Build history of the part. All positions in model axes, mm. Face numbers are marked on the shaded views. A direction names the side the tool comes from. Round coordinates to 2 decimals unless told otherwise and drop trailing zeros. Write each loop counter-clockwise with the first axis right and the second up, starting at its lowest first coordinate (ties: lowest second). Pieces come first, ordered by that corner, then holes. Notation, with made-up numbers: (-9, 12.5) -> (50, 12.5) arc R15 ccw to (50, 27.5) -> close; hole circle Ø9 at (57.25, 33.5). An arc over 180 degrees is marked (long way). Return JSON: item names as keys, results as strings.
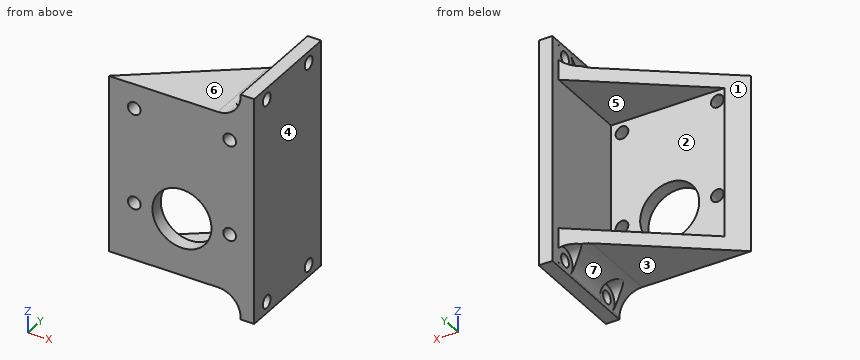
from build123d import *

# Parameters (mm, degrees)
EXTRUDE_1_DEPTH           = 39
SHELL_1_T                 = -3
SKETCH_2_R                = 1.4
CUT_EXTRUDE_1_DEPTH       = 30
SKETCH_3_R                = 6.5
CUT_EXTRUDE_2_DEPTH       = 5
SKETCH_5_W                = 50
SKETCH_5_H                = 24
EXTRUDE_2_DEPTH           = 3
SKETCH_4_R                = 1.4
CUT_EXTRUDE_3_DEPTH       = 5
FILLET_1_R                = 5
CUT_EXTRUDE_4_OUTLINE_R   = 1.4
CUT_EXTRUDE_4_OUTLINE_R_2 = 2.75
CUT_EXTRUDE_4_DEPTH       = 3.43874985


with BuildPart() as part:
    # ｽｹｯﾁ1 → ﾎﾞｽ - 押し出し1 (new body)
    with BuildSketch(Plane.XY):
        Polygon((0, 0), (32, 0), (32, 24), align=None)
    extrude(amount=EXTRUDE_1_DEPTH)

    # ｼｪﾙ1
    shell_1_openings = [part.faces().sort_by_distance(p)[0] for p in [
        (16, 12, 19.5),
    ]]
    offset(amount=SHELL_1_T, openings=shell_1_openings, kind=Kind.INTERSECTION)

    # ｽｹｯﾁ2 → ｶｯﾄ - 押し出し1 (cut)
    with BuildSketch(Plane.XZ):
        with Locations(Location((26.6, 12.609, 0), (0, 0, 270))):
            Circle(SKETCH_2_R)
        with Locations(Location((5.6, 12.609, 0), (0, 0, 270))):
            Circle(SKETCH_2_R)
        with Locations(Location((5.6, 33.609, 0), (0, 0, 270))):
            Circle(SKETCH_2_R)
        with Locations(Location((26.6, 33.609, 0), (0, 0, 270))):
            Circle(SKETCH_2_R)
    extrude(amount=-CUT_EXTRUDE_1_DEPTH, mode=Mode.SUBTRACT)

    # ｽｹｯﾁ3 → ｶｯﾄ - 押し出し2 (cut)
    with BuildSketch(Plane.XZ):
        with Locations(Location((16.1, 12.609, 0), (0, 0, 270))):
            Circle(SKETCH_3_R)
    extrude(amount=-CUT_EXTRUDE_2_DEPTH, mode=Mode.SUBTRACT)

    # ｽｹｯﾁ5 → ﾎﾞｽ - 押し出し2 (add)
    with BuildSketch(Plane(origin=(32, 0, 0), x_dir=(0, 0, -1), z_dir=(1, 0, 0))):
        with Locations((-19.5, 12)):
            Rectangle(SKETCH_5_W, SKETCH_5_H)
    extrude(amount=-EXTRUDE_2_DEPTH)

    # ｽｹｯﾁ4 → ｶｯﾄ - 押し出し3 (cut)
    with BuildSketch(Plane(origin=(32, 0, 0), x_dir=(0, 0, -1), z_dir=(1, 0, 0))):
        with Locations((3, 19.5)):
            Circle(SKETCH_4_R)
        with Locations((-42, 19.5)):
            Circle(SKETCH_4_R)
        with Locations((-42, 4.5)):
            Circle(SKETCH_4_R)
        with Locations((3, 4.5)):
            Circle(SKETCH_4_R)
    extrude(amount=-CUT_EXTRUDE_3_DEPTH, mode=Mode.SUBTRACT)

    # ﾌｨﾚｯﾄ1
    # the kernel refuses this fillet: 5 mm, written as the material it adds along each edge
    with BuildSketch(Plane(origin=(29, 34.25, 39), x_dir=(-1, 0, 0), z_dir=(0, -1, 0))) as fillet_1_piece_1_section:
        with BuildLine():
            CenterArc((FILLET_1_R, -FILLET_1_R), FILLET_1_R, 90, 90)
            Line((0, -FILLET_1_R), (0, 0))
            Line((0, 0), (FILLET_1_R, 0))
        make_face()
    fillet_1_piece_1 = extrude(amount=34.25, mode=Mode.PRIVATE)
    fillet_1_piece_1 = split(fillet_1_piece_1, bisect_by=Plane(origin=(35, 26.25, 39), z_dir=(0.6, -0.8, 0)), keep=Keep.TOP, mode=Mode.PRIVATE)
    fillet_1_piece_1 = fillet_1_piece_1 - Plane(origin=(29, 4.5, 42), x_dir=(0, 0, -1), z_dir=(1, 0, 0)) * Cylinder(1.4, 89, mode=Mode.PRIVATE)
    fillet_1_piece_1 = fillet_1_piece_1 - Plane(origin=(29, 19.5, 42), x_dir=(0, 0, -1), z_dir=(1, 0, 0)) * Cylinder(1.4, 89, mode=Mode.PRIVATE)
    add(fillet_1_piece_1)
    with BuildSketch(Plane(origin=(29, 34.25, 0), x_dir=(-1, 0, 0), z_dir=(0, -1, 0))) as fillet_1_piece_2_section:
        with BuildLine():
            CenterArc((FILLET_1_R, FILLET_1_R), FILLET_1_R, 180, 90)
            Line((0, FILLET_1_R), (0, 0))
            Line((0, 0), (FILLET_1_R, 0))
        make_face()
    fillet_1_piece_2 = extrude(amount=34.25, mode=Mode.PRIVATE)
    fillet_1_piece_2 = split(fillet_1_piece_2, bisect_by=Plane(origin=(35, 26.25, 0), z_dir=(0.6, -0.8, 0)), keep=Keep.TOP, mode=Mode.PRIVATE)
    fillet_1_piece_2 = fillet_1_piece_2 - Plane(origin=(29, 4.5, -3), x_dir=(0, 0, -1), z_dir=(1, 0, 0)) * Cylinder(1.4, 89, mode=Mode.PRIVATE)
    fillet_1_piece_2 = fillet_1_piece_2 - Plane(origin=(29, 19.5, -3), x_dir=(0, 0, -1), z_dir=(1, 0, 0)) * Cylinder(1.4, 89, mode=Mode.PRIVATE)
    add(fillet_1_piece_2)

    # ｶｯﾄ - 押し出し4: read off the stored shape, not the designer's step
    # ｶｯﾄ - 押し出し4 outline → ｶｯﾄ - 押し出し4 (cut)
    # profile 1 of 4: a face of its own
    with BuildSketch(Plane.ZY.offset(-29)):
        with BuildLine():
            ThreePointArc((44, 17.612541391), (44.75, 19.5), (44, 21.387458609))
            ThreePointArc((44, 21.387458609), (43.799721616, 21.579303274), (43.58113883, 21.75))
            ThreePointArc((43.58113883, 21.75), (42, 22.25), (40.41886117, 21.75))
            ThreePointArc((40.41886117, 21.75), (39.920696726, 17.700278384), (44, 17.612541391))
        make_face()
        with Locations((42, 19.5)):
            Circle(CUT_EXTRUDE_4_OUTLINE_R, mode=Mode.SUBTRACT)
    # profile 2 of 4: a face of its own
    with BuildSketch(Plane.ZY.offset(-29)):
        with BuildLine():
            ThreePointArc((44, 2.612541391), (44.75, 4.5), (44, 6.387458609))
            ThreePointArc((44, 6.387458609), (39.25, 4.5), (44, 2.612541391))
        make_face()
        with Locations((42, 4.5)):
            Circle(CUT_EXTRUDE_4_OUTLINE_R, mode=Mode.SUBTRACT)
    # profile 3 of 4: a face of its own
    with BuildSketch(Plane.ZY.offset(-29)):
        with BuildLine():
            ThreePointArc((-5, 21.387458609), (-1.200278384, 17.420696726), (-4.58113883, 21.75))
            ThreePointArc((-4.58113883, 21.75), (-4.799721616, 21.579303274), (-5, 21.387458609))
        make_face()
        with Locations((-3, 19.5)):
            Circle(CUT_EXTRUDE_4_OUTLINE_R, mode=Mode.SUBTRACT)
    # profile 4 of 4: a face of its own
    with BuildSketch(Plane.ZY.offset(-29)):
        with Locations((-3, 4.5)):
            Circle(CUT_EXTRUDE_4_OUTLINE_R_2)
        with Locations((-3, 4.5)):
            Circle(CUT_EXTRUDE_4_OUTLINE_R, mode=Mode.SUBTRACT)
    extrude(amount=CUT_EXTRUDE_4_DEPTH, mode=Mode.SUBTRACT)


solid = part.part
Q1. Saw through at C-C on z = 4. List the corners of the cut face in (x, y), then the cut area to 3 significant figures.
Verdict:
{"outline": "(0, 0) -> (32, 0) -> (32, 24) -> (29, 24) -> (29, 3) -> (4, 3) -> close", "area": "153 mm²"}
Q2. Saw through at D-D on y = 15. List the corners of the cut face in (x, z).
Verdict:
{"outline": "(20, 0) -> (24, 0) arc R5 cw to (29, -5) -> (29, -5.5) -> (32, -5.5) -> (32, 44.5) -> (29, 44.5) -> (29, 44) arc R5 cw to (24, 39) -> (20, 39) -> (20, 36) -> (29, 36) -> (29, 3) -> (20, 3) -> close"}
Q3. Saw through at B-B on y = 4.5. List the corners of the cut face in (x, z).
Verdict:
{"outline": "(6, 0) -> (24, 0) arc R5 cw to (25.56, -0.25) -> (29, -0.25) -> (29, -1.6) -> (32, -1.6) -> (32, 40.6) -> (29, 40.6) -> (29, 39.25) -> (25.56, 39.25) arc R5 cw to (24, 39) -> (6, 39) -> (6, 36) -> (29, 36) -> (29, 3) -> (6, 3) -> close; (29, -5.5) -> (32, -5.5) -> (32, -4.4) -> (29, -4.4) -> close; (29, 43.4) -> (32, 43.4) -> (32, 44.5) -> (29, 44.5) -> close"}
Q4. 3-axis set-ups, long thin cutter, end or side, ignore diameter. For the marked faces 1, 2 and 3: which of +Z, -Z, +X, -X, +Y, -Y reach the whole face in a straight line?
Verdict:
{"face 1": "+Z, -Z, -X, +Y", "face 2": "-X, +Y", "face 3": "-Z, -X, +Y, -Y"}
Q5. Two-plate mould, pull along Z, no slides. Class the marked faces 4, 5, 6 and 7: +Z half, -Z half, draft (parallel to the pull), parting line (faces both ways), or undercut.
Verdict:
{"face 4": "draft", "face 5": "undercut", "face 6": "+Z half", "face 7": "-Z half"}
Q6. Saw through at A-A on x = 5.6. List the corners of the cut face in (y, z).
Verdict:
{"outline": "(0, 0) -> (4.2, 0) -> (4.2, 3) -> (3, 3) -> (3, 11.21) -> (0, 11.21) -> close; (0, 14.01) -> (3, 14.01) -> (3, 32.21) -> (0, 32.21) -> close; (0, 35.01) -> (3, 35.01) -> (3, 36) -> (4.2, 36) -> (4.2, 39) -> (0, 39) -> close"}
Q7. Pin check, flat tips, straight feed: pin 1 Ø5.5 at (x, y) = (20.5, 12) entering from +Z; pin 2 Ø4.5 at (y, z) = (4.5, 42) entering from -X; pin 3 Ø8 at (x, y) = (15, 3.5) entering from -Z. Stop position of each tip, or through.
Verdict:
{"pin 1": "stops at z = 39", "pin 2": "stops at x = 29", "pin 3": "stops at z = 0"}
Q8. Wall check: L1, parallel to Z at x = 27.6, y = 4.5; L2, parallel to Z at x = 24, y = 5.5; L3, parallel to X at y = 11.5, z = 27. Give the ranges that are in metal, low to high.
Verdict:
{"L1": "z = -0.25 to 3, 36 to 39.25", "L2": "z = 0 to 3, 36 to 39", "L3": "x = 29 to 32"}
